from build123d import *

# Parameters (mm, degrees)
F0_W      = 6.35
F0_H      = 203.5342199714
F1_DEPTH  = 101.6
F2_W      = 101.6
F2_H      = 6.35
F3_DEPTH  = 25.4
F5_W      = 12.7
F5_H      = 12.7
F6_DEPTH  = 254
F7_R      = 1.905
F8_DEPTH  = 25.4
F9_W      = 12.7
F9_H      = 12.7
F10_DEPTH = 50.8


with BuildPart() as f1:
    # F0 (on Right) → F1 (new body)
    with BuildSketch(Plane.YZ):
        Polygon((-3.0652988178, -75.2811529749), (-98.3152988178, -75.2811529749), (-98.3152988178, -81.6311529749), (3.2847011822, -81.6311529749), (3.2847011822, -75.2811529749), align=None)
        with Locations((0.1097011822, 26.4859570108)):
            Rectangle(F0_W, F0_H)
    extrude(amount=F1_DEPTH)

    # F2 (on face) → F3 (join)
    with BuildSketch(Plane.XY.offset(-75.2811529749)):
        with Locations((50.8, -95.1402988178)):
            Rectangle(F2_W, F2_H)
    extrude(amount=F3_DEPTH)


with BuildPart() as f6:
    # F5 (on Top) → F6 (new body)
    with BuildSketch(Plane.XY):
        with Locations((-32.7810319141, 16.882541026)):
            Rectangle(F5_W, F5_H)
    extrude(amount=F6_DEPTH)

    # F7 (on face) → F8 (cut)
    with BuildSketch(Plane.XY.offset(254)):
        with Locations((-32.7810319141, 16.882541026)):
            Circle(F7_R)
    extrude(amount=-F8_DEPTH, mode=Mode.SUBTRACT)

    # F9 (on face) → F10 (join)
    with BuildSketch(Plane.XZ.offset(-10.532541026)):
        with Locations((-32.7810319141, 6.35)):
            Rectangle(F9_W, F9_H)
    extrude(amount=F10_DEPTH)


solid = f6.part
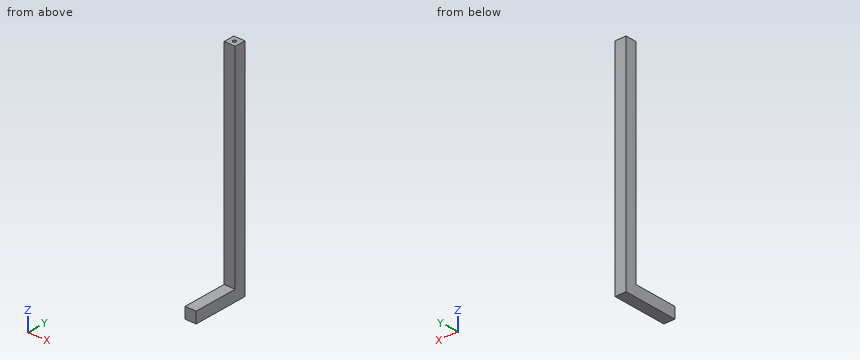
Input: part model. Units: mm. Frame: model coordinates. Round coordinates to 2 decimals unless told otherwise and drop trailing zeros. Write each loop counter-clockwise with the first axis right and the second up, starting at its lowest first coordinate (ties: lowest second). Pieces come first, ordered by that corner, then holes.
1) Cut plane A-A (x = -37). Return the cut outline in (y, z).
2) Cut plane C-C (y = -20). Return the cut outline in (x, z), then the cut area to 3 significant figures.
3) Contact query for flat-ended pins moving along their axis: P1, Ø3, axis at x = -32.5, y = -32, coming from the +Z side; P2, Ø6.5, axis at x = -30, z = 141.5, coming from the -Y side. Output: stop coordinate, or through.
4) Cut plane B-B (z = 95). Return the cut outline in (x, y).
5) Ray query, L1, parallel to Z at x = -34.25, y = -19; L2, parallel to Y at x = -38, z = 82. Return the intervals inside material, ascending.
Geometry says:
1. outline: (-40.27, 0) - (23.23, 0) - (23.23, 254) - (10.53, 254) - (10.53, 12.7) - (-40.27, 12.7) - close
2. outline: (-39.13, 0) - (-26.43, 0) - (-26.43, 12.7) - (-39.13, 12.7) - close
2. area: 161 mm2
3. P1: stops at z = 12.7
3. P2: stops at y = 10.53
4. outline: (-39.13, 10.53) - (-26.43, 10.53) - (-26.43, 23.23) - (-39.13, 23.23) - close
5. L1: z = 0 to 12.7
5. L2: y = 10.53 to 23.23
